Work out the finished part from the listing and answer in its coordinate system (mm). A direction names the side the tool comes from. Coordinates: 2 decimals unless noted, no trailing zeros. Order: outer loops, then holes, each group sorted by start corner. A loop starts at its lowest first (then second) coordinate and runs counter-clockwise, first axis right, second up.
```python
from build123d import *

# Parameters (mm, degrees)
HIP_BASE_EXTRUDED_BOSS_BASE_DEPTH      = 7.05
SKETCH1_3_R                            = 3.5
LEG_JOINT_EXTRUDED_BOSS_BASE_DEPTH     = 0.75
SKETCH2_R                              = 1.2
LEG_PEG_EXTRUDED_BOSS_BASE_DEPTH       = 2.4
LEG_PEG_INNER_EXTRUDED_BOSS_BASE_DEPTH = 1.2
LEG_LOCK_EXTRUDED_DETAIL_DEPTH         = 0.7
HIP_PEG_EXTRUDED_BOSS_BASE_DEPTH       = 4.8
HIP_CAVITY_EXTRUDED_CUT_DEPTH          = 4.8
HIP_PEG_CHAMFER_DEPTH                  = 12.495760088


with BuildPart() as part:
    # Sketch1 → Hip Base - Extruded Boss/Base (new, symmetric)
    with BuildSketch(Plane(origin=(0, 0, 0), x_dir=(0, 0, -1), z_dir=(1, 0, 0))):
        with BuildLine():
            ThreePointArc((-2.351256126, -2.107396168), (0, -1.2), (2.351256126, -2.107396168))
            Line((2.351256126, -2.107396168), (3.9, -2.107396168))
            Line((3.9, -2.107396168), (3.9, -0.007396168))
            Line((3.9, -0.007396168), (-3.9, -0.007396168))
            Line((-3.9, -0.007396168), (-3.9, -2.107396168))
            Line((-3.9, -2.107396168), (-2.351256126, -2.107396168))
        make_face()
    extrude(amount=HIP_BASE_EXTRUDED_BOSS_BASE_DEPTH, both=True)

    # Sketch1<3> → Leg Joint - Extruded Boss/Base (add, symmetric)
    with BuildSketch(Plane(origin=(0, 0, 0), x_dir=(0, 0, -1), z_dir=(1, 0, 0))):
        with Locations((0, -4.7)):
            Circle(SKETCH1_3_R)
    extrude(amount=LEG_JOINT_EXTRUDED_BOSS_BASE_DEPTH, both=True)

    # Sketch2 → Leg Peg - Extruded Boss/Base (add)
    with BuildSketch(Plane(origin=(0.75, 0, 0), x_dir=(0, 0, -1), z_dir=(1, 0, 0))):
        with Locations((0, -4.7)):
            Circle(SKETCH2_R)
    leg_peg_extruded_boss_base = extrude(amount=LEG_PEG_EXTRUDED_BOSS_BASE_DEPTH)

    # Sketch3 → Leg Peg Inner - Extruded Boss/Base (add)
    with BuildSketch(Plane(origin=(3.15, 0, 0), x_dir=(0, 0, -1), z_dir=(1, 0, 0))):
        with BuildLine():
            Line((-0.661437828, -3.95), (0.661437828, -3.95))
            ThreePointArc((0.661437828, -3.95), (0, -5.7), (-0.661437828, -3.95))
        make_face()
    leg_peg_inner_extruded_boss_base = extrude(amount=LEG_PEG_INNER_EXTRUDED_BOSS_BASE_DEPTH)

    # Sketch4 → Leg Lock - Extruded Detail (add)
    with BuildSketch(Plane(origin=(3.15, 0, 0), x_dir=(0, 0, -1), z_dir=(1, 0, 0))):
        with BuildLine():
            Line((-0.7, -5.8892855), (-0.7, -5.414142843))
            ThreePointArc((-0.7, -5.414142843), (0, -5.7), (0.7, -5.414142843))
            Line((0.7, -5.414142843), (0.7, -5.8892855))
            ThreePointArc((0.7, -5.8892855), (0, -6.08), (-0.7, -5.8892855))
        make_face()
    leg_lock_extruded_detail = extrude(amount=LEG_LOCK_EXTRUDED_DETAIL_DEPTH)

    # Sketch5 → Hip Peg - Extruded Boss/Base (add)
    with BuildSketch(Plane(origin=(0, -0.007396168, 0), x_dir=(1, 0, 0), z_dir=(0, 1, 0))):
        with BuildLine():
            ThreePointArc((1.55, -1), (2.539949494, -1.410050506), (2.95, -2.4))
            Line((2.95, -2.4), (4.95, -2.4))
            ThreePointArc((4.95, -2.4), (5.360050506, -1.410050506), (6.35, -1))
            Line((6.35, -1), (6.35, 1))
            ThreePointArc((6.35, 1), (5.360050506, 1.410050506), (4.95, 2.4))
            Line((4.95, 2.4), (2.95, 2.4))
            ThreePointArc((2.95, 2.4), (2.539949494, 1.410050506), (1.55, 1))
            Line((1.55, 1), (1.55, -1))
        make_face()
    hip_peg_extruded_boss_base = extrude(amount=HIP_PEG_EXTRUDED_BOSS_BASE_DEPTH)

    # Sketch6 → Hip Cavity - Extruded Cut (cut)
    with BuildSketch(Plane(origin=(0, 4.792603832, 0), x_dir=(1, 0, 0), z_dir=(0, 1, 0))):
        with BuildLine():
            Line((5.058021727, -0.855738191), (5.05, 0.866025404))
            ThreePointArc((5.05, 0.866025404), (2.550015194, -0.006522554), (5.058021727, -0.855738191))
        make_face()
    hip_cavity_extruded_cut = extrude(amount=-HIP_CAVITY_EXTRUDED_CUT_DEPTH, mode=Mode.SUBTRACT)

    # Sketch7 → Hip Peg Chamfer (cut, symmetric)
    with BuildSketch(Plane.XY):
        Polygon((6.35, 4.792603832), (6.35, 1.792603832), (5.85, 4.792603832), align=None)
    hip_peg_chamfer = extrude(amount=HIP_PEG_CHAMFER_DEPTH, both=True, mode=Mode.SUBTRACT)

    # Mirror1: Leg Peg - Extruded Boss/Base, Leg Peg Inner - Extruded Boss/Base, Leg Lock - Extruded Detail, Hip Peg - Extruded Boss/Base, Hip Cavity - Extruded Cut, Hip Peg Chamfer across plane
    add(leg_peg_extruded_boss_base.mirror(Plane(origin=(0, 0, 0), x_dir=(0, 0, 1), z_dir=(1, 0, 0))))
    add(leg_peg_inner_extruded_boss_base.mirror(Plane(origin=(0, 0, 0), x_dir=(0, 0, 1), z_dir=(1, 0, 0))))
    add(leg_lock_extruded_detail.mirror(Plane(origin=(0, 0, 0), x_dir=(0, 0, 1), z_dir=(1, 0, 0))))
    add(hip_peg_extruded_boss_base.mirror(Plane(origin=(0, 0, 0), x_dir=(0, 0, 1), z_dir=(1, 0, 0))))
    add(hip_cavity_extruded_cut.mirror(Plane(origin=(0, 0, 0), x_dir=(0, 0, 1), z_dir=(1, 0, 0))), mode=Mode.SUBTRACT)
    add(hip_peg_chamfer.mirror(Plane(origin=(0, 0, 0), x_dir=(0, 0, 1), z_dir=(1, 0, 0))), mode=Mode.SUBTRACT)


solid = part.part
```
1. The part is cut by section C-C (y = -4.7). Determine the outline of the cut face in (x, z).
2. Consider probe 1 along X at (y, z) = (1.5, 0); probe 2 along Z at (x, y) = (3.95, 3.6); probe 3 along X at (y, z) = (1.95, 0). Determine where each line is inside the solid, lowest interval first.
3. The part is cut by section A-A (y = 2). Determine the outline of the cut face in (x, z).
4. The mould has two halves that part along Z. Classify faces 6 (the cylindrical face through (-3.9, -1.2, 0)), 7 (the flat face through (-4, 2, -2.4)), 8 (the flat face through (4, 2, 2.4)): released by +Z, released by -Z, zero draft, split by the parting line, or undercut.
5. The part is cut by section B-B (x = 1.75). Determine the outline of the cut face in (y, z).
6. Flat-ended cylindrical pins translate along their axes: pin 1 (3 mm diameter, centred on x = 0.5, z = 2, fed in from -Y); pin 2 (1 mm diameter, centred on x = 4, z = 0, fed in from +Y); pin 3 (1.5 mm diameter, centred on x = -1, z = -1.5, fed in from -Y); pin 4 (1 mm diameter, centred on x = 0, y = 2, fed in from +Z). Find the tip coordinate at first contact, or state that the pin passes through.
7. For faces 1 (the flat face through (4, 2, -2.4)), 2 (the flat face through (1.55, 2, 0)), 3 (the cylindrical face through (2.53, 2.36, 1.4)), 4 (the flat face through (-4, 2, 2.4)), 5 (the cylindrical face through (-4, -5.7, 0)), determine the directions among +Z, -Z, +X, -X, +Y, -Y from which every point of the face is accessible in a straight line to the end or side of a thin tool.
8. The part is cut by section D-D (x = 0.25). Determine the outline of the cut face in (y, z).
Worked out:
1. outline: (-4.35, -1) - (-3.15, -1) - (-3.15, -1.2) - (-0.75, -1.2) - (-0.75, -3.5) - (0.75, -3.5) - (0.75, -1.2) - (3.15, -1.2) - (3.15, -1) - (4.35, -1) - (4.35, 1) - (3.15, 1) - (3.15, 1.2) - (0.75, 1.2) - (0.75, 3.5) - (-0.75, 3.5) - (-0.75, 1.2) - (-3.15, 1.2) - (-3.15, 1) - (-4.35, 1) - close
2. probe 1: x = -6.35 to -5.05, -2.55 to -1.55, 1.55 to 2.55, 5.05 to 6.35
2. probe 2: z = -2.4 to -1.4, 1.4 to 2.4
2. probe 3: x = -6.32 to -5.05, -2.55 to -1.55, 1.55 to 2.55, 5.05 to 6.32
3. outline: (-6.32, -1) arc R1.4 cw to (-4.95, -2.4) - (-2.95, -2.4) arc R1.4 cw to (-1.55, -1) - (-1.55, 1) arc R1.4 cw to (-2.95, 2.4) - (-4.95, 2.4) arc R1.4 cw to (-6.32, 1) - close; (1.55, -1) arc R1.4 cw to (2.95, -2.4) - (4.95, -2.4) arc R1.4 cw to (6.32, -1) - (6.32, 1) arc R1.4 cw to (4.95, 2.4) - (2.95, 2.4) arc R1.4 cw to (1.55, 1) - close; hole (-5.06, 0.86) - (-5.05, -0.87) arc R1.4 ccw (long way) to start; hole (5.05, -0.87) - (5.06, 0.86) arc R1.4 ccw (long way) to start
4. face 6: undercut
4. face 7: released by -Z
4. face 8: released by +Z
5. outline: circle Ø2.4 at (-4.7, 0); (-2.11, -3.9) - (-0.01, -3.9) - (-0.01, -1.01) - (4.79, -1.01) - (4.79, 1.01) - (-0.01, 1.01) - (-0.01, 3.9) - (-2.11, 3.9) - (-2.11, 2.35) arc R3.5 cw to (-2.11, -2.35) - close
6. pin 1: stops at y = -8.16
6. pin 2: stops at y = -0.01
6. pin 3: stops at y = -8.11
6. pin 4: passes through
7. face 1: -Z, +X, -X, +Y
7. face 2: +Z, -Z, +Y
7. face 3: +Z, +Y
7. face 4: +Z, +X, -X, +Y
7. face 5: -X
8. outline: (-2.11, -3.9) - (-0.01, -3.9) - (-0.01, 3.9) - (-2.11, 3.9) - (-2.11, 2.35) arc R3.5 ccw (long way) to (-2.11, -2.35) - close
